Part print with two shaded views. Sizes in mm from the minimum x, y, z corner. A direction names the side the tool comes from. Round coordinates to 2 decimals unless told otherwise and drop trailing zeros. Write each loop counter-clockwise with the first axis right and the second up, starting at its lowest first coordinate (ties: lowest second). Pieces come first, ordered by that corner, then holes. Notation, with made-up numbers: (30, 80) - (41, 80) arc R17 ccw to (41, 102) - close; hole circle Ø4 at (8.5, 79.25). An arc over 180 degrees is marked (long way). Answer as a JSON object with one key per item and string values. Group by question number.
Item 1: Which spindle directions (+Z, -Z, +X, -X, +Y, -Y) get a long thin tool onto all of the face, cutting with end or side? Do the marked faces 4 and 5. Say none if no direction does.
Item 2: Slice it at A-A, the plane z = 196.5. List the corners of the cut face in (x, y), then the cut area to 3 significant figures.
Item 3: Slice it at D-D, the plane z = 116.5. List the corners of the cut face in (x, y), then the cut area to 3 significant figures.
Item 4: Slice it at C-C, the plane y = 105.5. List the corners of the cut face in (x, z).
Item 5: Probe line 1 (X direction, y = 109.5, z = 161.5); line 2 (Z direction, x = 140.5, y = 20); line 3 (X direction, y = 5, z = 239). List the from-to ranges inside material, lowest first. Write a range as from..to.
Item 6: Slice it at B-B, the plane x = 200. List the corners of the cut face in (y, z), then the cut area to 3 significant figures.
Item 7: Flat gauge pin, fed straight in: pin 1 (3 mm diameter, centred on x = 33.5, z = 307, fed in from +Y). Where does the tip first touch, or does it go through?
Item 8: Two-plate mould, pull along X, no slides. Class the marked faces 1, 2 and 3: +X half, -X half, draft (parallel to the pull), parting line (faces both ways), or undercut.
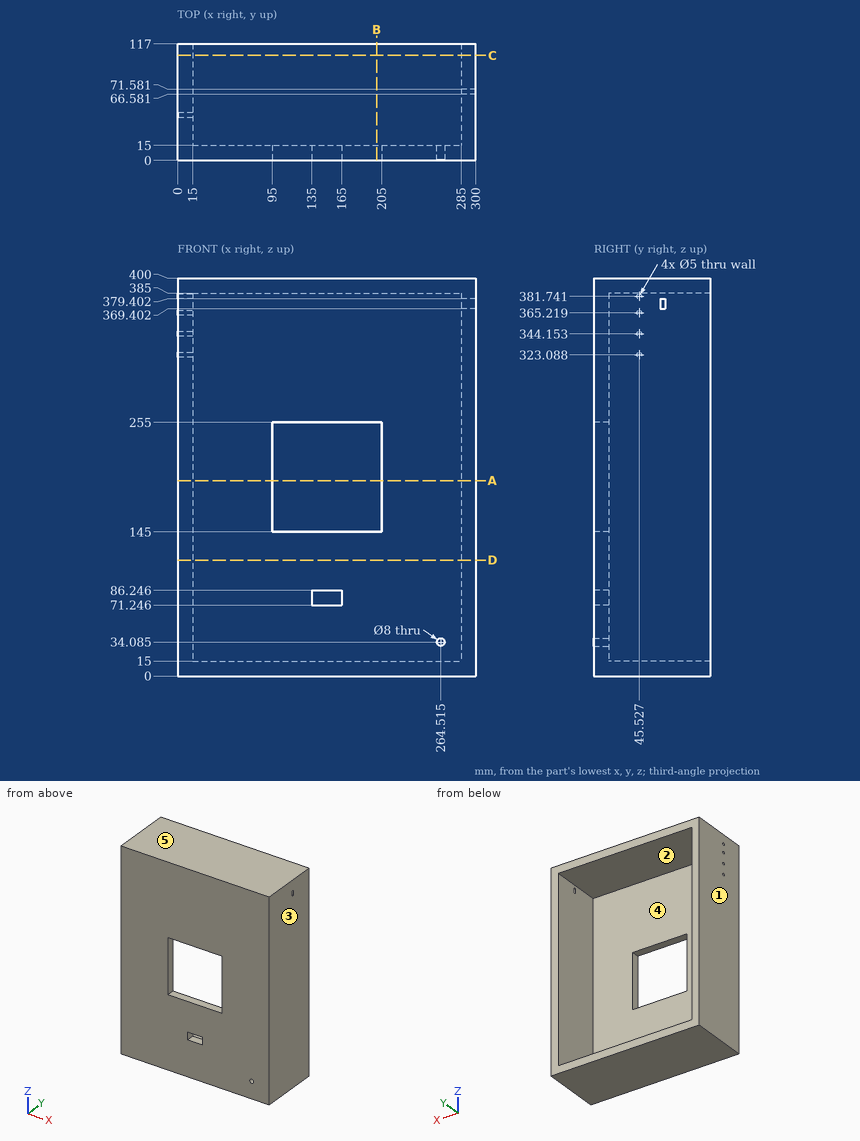
Geometry says:
{
 "1": {"face 4": "+Y", "face 5": "+Z, +X, -X, +Y, -Y"},
 "2": {"outline": "(0, 0) - (95, 0) - (95, 15) - (15, 15) - (15, 117) - (0, 117) - close; (205, 0) - (300, 0) - (300, 117) - (285, 117) - (285, 15) - (205, 15) - close", "area": "5,910 mm^2"},
 "3": {"outline": "(0, 0) - (300, 0) - (300, 117) - (285, 117) - (285, 15) - (15, 15) - (15, 117) - (0, 117) - close", "area": "7,560 mm^2"},
 "4": {"outline": "(0, 0) - (300, 0) - (300, 400) - (0, 400) - close; hole (15, 15) - (285, 15) - (285, 385) - (15, 385) - close"},
 "5": {"line 1": "x = 0..15, 285..300", "line 2": "z = 0..15, 385..400", "line 3": "x = 0..95, 205..300"},
 "6": {"outline": "(0, 0) - (117, 0) - (117, 15) - (15, 15) - (15, 145) - (0, 145) - close; (0, 255) - (15, 255) - (15, 385) - (117, 385) - (117, 400) - (0, 400) - close", "area": "7,410 mm^2"},
 "7": {"pin 1": "stops at y = 15"},
 "8": {"face 1": "-X half", "face 2": "undercut", "face 3": "+X half"}
}
